Part model, mm, in its own coordinate system. Face numbers are marked on the shaded views. A direction names the side the tool comes from. Coordinates: 2 decimals unless noted, no trailing zeros. Loops run counter-clockwise (first coordinate to the right, second up) from the corner with the lowest first, then second, coordinate; pieces in that order, holes last. Notation, with made-up numbers: M 22,-19 L 55,-19 A15 cw 55,1 Z; hole C -23.5,-24.5 d11. An arc over 180 degrees is marked long. Use CSV: the item, a comma, the result in double quotes. Start each with the question number.
from build123d import *
from build123d.topology import SkipClean

# Parameters (mm, degrees)
SKETCH1_R           = 8
BOSS_EXTRUDE1_DEPTH = 1
SKETCH2_R           = 6
BOSS_EXTRUDE2_DEPTH = 2.5
BOSS_EXTRUDE2_TAPER = 45
SKETCH3_R           = 3.5
BOSS_EXTRUDE3_DEPTH = 4
SKETCH4_R           = 3.5
BOSS_EXTRUDE4_DEPTH = 1
BOSS_EXTRUDE4_DRAFT = -59
SKETCH6_R           = 5.164279482
BOSS_EXTRUDE5_DEPTH = 1
SKETCH7_R           = 6.5
BOSS_EXTRUDE6_DEPTH = 3
SKETCH9_R           = 8
SKETCH9_R_2         = 7
BOSS_EXTRUDE7_DEPTH = 1
SKETCH10_R          = 1.4
CUT_EXTRUDE1_DEPTH  = 6


with BuildPart() as part:
    # Sketch1 → Boss-Extrude1 (new body)
    with BuildSketch(Plane(origin=(0, 0, 0), x_dir=(1, 0, 0), z_dir=(0, 1, 0))):
        with Locations(Location((0, 0, 0), (0, 0, 270))):
            Circle(SKETCH1_R)
    extrude(amount=BOSS_EXTRUDE1_DEPTH)

    # Sketch2 → Boss-Extrude2 (add)
    with BuildSketch(Plane(origin=(0, 1, 0), x_dir=(1, 0, 0), z_dir=(0, 1, 0))):
        Circle(SKETCH2_R)
    extrude(amount=BOSS_EXTRUDE2_DEPTH, taper=BOSS_EXTRUDE2_TAPER)

    # Sketch3 → Boss-Extrude3 (add)
    with BuildSketch(Plane(origin=(0, 3.5, 0), x_dir=(1, 0, 0), z_dir=(0, 1, 0))):
        with Locations(Location((0, 0, 0), (0, 0, 270))):
            Circle(SKETCH3_R)
    extrude(amount=BOSS_EXTRUDE3_DEPTH)


with BuildPart() as boss_extrude4_tool:
    # Sketch4 → Boss-Extrude4 (with draft: the straight prism first)
    with BuildSketch(Plane(origin=(0, 7.5, 0), x_dir=(1, 0, 0), z_dir=(0, 1, 0))):
        with Locations(Location((0, 0, 0), (0, 0, 270))):
            Circle(SKETCH4_R)
    extrude(amount=BOSS_EXTRUDE4_DEPTH)
    # Boss-Extrude4: the draft: its side faces are tilted about the plane it starts from
    boss_extrude4_sides = [boss_extrude4_tool.faces().sort_by_distance(p)[0] for p in [
        (0, 8, -3.5),
    ]]
    draft(boss_extrude4_sides, Plane(origin=(0, 7.5, 0), x_dir=(1, 0, 0), z_dir=(0, 1, 0)), BOSS_EXTRUDE4_DRAFT)


with BuildPart() as part_1:
    add(part.part)

    # Boss-Extrude4: add boss_extrude4_tool
    add(boss_extrude4_tool.part)

    # Sketch6 → Boss-Extrude5 (add)
    with BuildSketch(Plane(origin=(0, 8.5, 0), x_dir=(1, 0, 0), z_dir=(0, 1, 0))):
        with Locations(Location((0, 0, 0), (0, 0, 270))):
            Circle(SKETCH6_R)
    extrude(amount=BOSS_EXTRUDE5_DEPTH)

    # Sketch7 → Boss-Extrude6 (add)
    with BuildSketch(Plane(origin=(0, 9.5, 0), x_dir=(1, 0, 0), z_dir=(0, 1, 0))):
        with Locations(Location((0, 0, 0), (0, 0, 270))):
            Circle(SKETCH7_R)
    extrude(amount=BOSS_EXTRUDE6_DEPTH)

    # Sketch8 → Revolve1 (revolve)
    with SkipClean():  # the faces are left unmerged after this step: merging them gives an invalid solid
        with BuildSketch(Plane.XY):
            with BuildLine():
                ThreePointArc((-0.12, 15.075463153), (-3.329649921, 14.403365131), (-6, 12.5))
                Line((-6, 12.5), (-0.12, 12.5))
                Line((-0.12, 12.5), (-0.12, 15.075463153))
            make_face()
            with BuildLine():
                Line((-0.12, 15.075463153), (-0.12, 12.5))
                Line((-0.12, 12.5), (5.76, 12.5))
                ThreePointArc((5.76, 12.5), (3.089649921, 14.403365131), (-0.12, 15.075463153))
            make_face()
        revolve(axis=Axis((-0.12, 12.5, 0), (0, 1, 0)))
    add(part_1.part.scale(1), mode=Mode.REPLACE)  # the faces are merged on a copy

    # Sketch9 → Boss-Extrude7 (add)
    with BuildSketch(Plane(origin=(0, 1, 0), x_dir=(1, 0, 0), z_dir=(0, 1, 0))):
        with Locations(Location((0, 0, 0), (0, 0, 270))):
            Circle(SKETCH9_R)
        with Locations(Location((0, 0, 0), (0, 0, 270))):
            Circle(SKETCH9_R_2, mode=Mode.SUBTRACT)
    extrude(amount=BOSS_EXTRUDE7_DEPTH)

    # Sketch10 → Cut-Extrude1 (cut)
    with BuildSketch(Plane.XZ):
        with Locations(Location((0, 0, 0), (0, 0, 270))):
            Circle(SKETCH10_R)
    extrude(amount=-CUT_EXTRUDE1_DEPTH, mode=Mode.SUBTRACT)

    # Chamfer1: read off the stored shape, not the designer's step
    # Chamfer1 outline → Chamfer1 (revolve)
    with BuildSketch(Plane.XY):
        Polygon((5.164279482, 9.5), (5.164279482, 8.5), (5.915896622, 8.95161714), (6.464279482, 9.5), align=None)
    revolve(axis=Axis((0, 0, 0), (0, 1, 0)))


solid = part_1.part
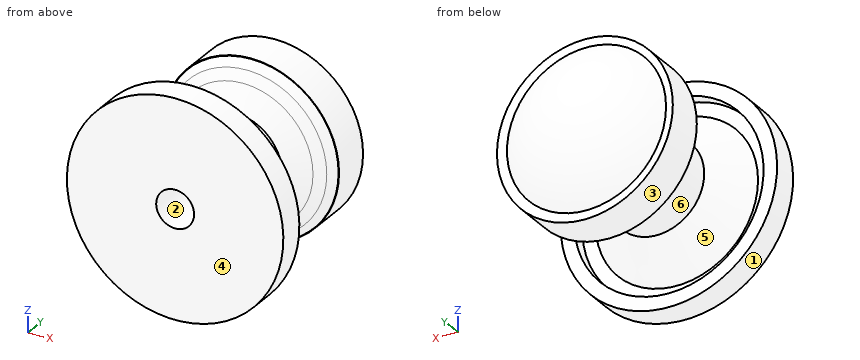
1. Slice it at A-A, the plane y = 10.25. List the corners of the cut face in (x, z).
2. Wall check: probe 1 along X at (y, z) = (1.2, 0); probe 2 along Z at (x, y) = (0.5, 1.75); probe 3 along Y at (x, z) = (3, 7.25). Give the ranges that are in metal, low to high.
3. Two-plate mould, pull along Y, no slides. Class the marked faces 3, 4, 5 and 6: pulls with the +Y half, pulls with the -Y half, needs draft (parallel to the pull), parting line crosses it, or undercut.
4. Tool access for the marked faces 1 and 2: list every direction of +Z, -Z, +X, -X, +Y, -Y with a clear straight run to the whole face (end or side of a thin tool).
5. Pin check, flat tips, straight feed: pin 1 (2 mm diameter, centred on x = 0.5, y = 8, fed in from +Z); pin 2 (2 mm diameter, centred on y = 10, z = -3.5, fed in from +X); pin 3 (1.4 mm diameter, centred on x = 0, z = 0, fed in from -Y). Stop position of each tip, or through.
6. Slice it at B-B, the plane y = 13.75. List the corners of the cut face in (x, z), and give its area (3 significant figures).
Found:
1,outline,"C 0,0 d13"
2,probe 1,"-8 to -7, -5.8 to -1.4, 1.4 to 5.8, 7 to 8"
2,probe 2,"-7.98 to -6.98, -5.23 to -1.31, 1.31 to 5.23, 6.98 to 7.98"
2,probe 3,"0 to 2"
3,face 3,"needs draft"
3,face 4,"pulls with the -Y half"
3,face 5,"undercut"
3,face 6,"undercut"
4,face 1,"+Y, -Y"
4,face 2,"-Y"
5,pin 1,"z = 5.95"
5,pin 2,"x = 6"
5,pin 3,"y = 6"
6,outline,"C -0.12,0 d8.82"
6,area,"61.1 mm^2"
